Design review of the part built by this model. Coordinates are the model's own, in mm. Face numbers are marked on the shaded views. A direction names the side the tool comes from. Coordinates: 2 decimals unless noted, no trailing zeros. Write each loop counter-clockwise with the first axis right and the second up, starting at its lowest first coordinate (ties: lowest second). Pieces come first, ordered by that corner, then holes. Notation, with made-up numbers: (42, -0.5) -> (61, -0.5) arc R27 cw to (61, 21.5) -> close; hole circle Ø3 at (74.5, 35). An arc over 180 degrees is marked (long way). Return JSON: item names as keys, results as strings. Group by question number.
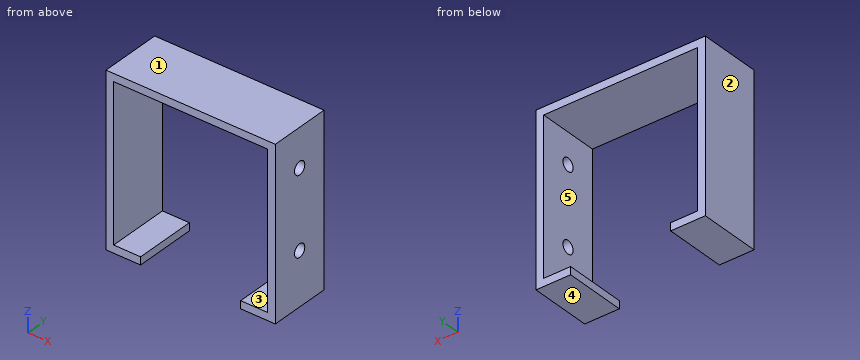
from build123d import *

# Parameters (mm, degrees)
BOSS_EXTRUDE1_DEPTH = 25.4
CUT_EXTRUDE1_REACH  = 71.85
SKETCH2_R           = 2.667


with BuildPart() as part:
    # Sketch1 → Boss-Extrude1 (new body)
    with BuildSketch(Plane(origin=(0, 0, 0), x_dir=(1, 0, 0), z_dir=(0, 1, 0))):
        Polygon((-3.175, -3.175), (-3.175, 63.5), (-3.175, 66.675), (11.1125, 66.675), (11.1125, 63.5), (0, 63.5), (0, 0), (63.5, 0), (63.5, 63.5), (52.3875, 63.5), (52.3875, 66.675), (66.675, 66.675), (66.675, 63.5), (66.675, -3.175), align=None)
    extrude(amount=BOSS_EXTRUDE1_DEPTH)

    # Sketch2 → Cut-Extrude1 (cut, up to next)
    with BuildSketch(Plane(origin=(66.675, 0, 0), x_dir=(0, 0, -1), z_dir=(1, 0, 0)), mode=Mode.PRIVATE) as cut_extrude1_sk1:
        with Locations((12.7, 12.7)):
            Circle(SKETCH2_R)
    cut_extrude1_tool1 = extrude(cut_extrude1_sk1.sketch, amount=-CUT_EXTRUDE1_REACH, mode=Mode.PRIVATE) & part.part
    add(cut_extrude1_tool1.solids().sort_by_distance((66.675, 12.7, -12.7))[0], mode=Mode.SUBTRACT)
    # Sketch2 → Cut-Extrude1 (cut, up to next)
    with BuildSketch(Plane(origin=(66.675, 0, 0), x_dir=(0, 0, -1), z_dir=(1, 0, 0)), mode=Mode.PRIVATE) as cut_extrude1_sk2:
        with Locations((44.7675, 12.7)):
            Circle(SKETCH2_R)
    cut_extrude1_tool2 = extrude(cut_extrude1_sk2.sketch, amount=-CUT_EXTRUDE1_REACH, mode=Mode.PRIVATE) & part.part
    add(cut_extrude1_tool2.solids().sort_by_distance((66.675, 12.7, -44.7675))[0], mode=Mode.SUBTRACT)


solid = part.part
Q1. For P1, Ø1.5, axis at x = 44, y = 20.5, coming from the -Z side, flat-tipped, find the tip position at first contact; note if it passes through.
Q2. For the marked faces 4 and 5, list the 3-axis set-ups (+Z, -Z, +X, -X, +Y, -Y) from which the entire face can be reached by the end or side of a thin tool; tool diameter is ignored.
Q3. We need section A-A on z = -23.5. Write out the cut boundary in (x, y) (3 decimals).
Q4. We need section C-C on y = 12.7. Write out the cut boundary in (x, z) (1 decimal), plus the area to 3 significant figures.
Q5. The part is to be moulded in two halves that separate along Z. For the marked faces 1, 2 and 3, say which applies: +Z half, -Z half, draft (parallel to the pull), parting line (faces both ways), or undercut.
Q6. We need section D-D on z = -12.7. Write out the cut boundary in (x, y) (3 decimals).
Q7. We need section B-B on x = 57. Write out the cut boundary in (y, z) (3 decimals), plus the area to 3 significant figures.
Q8. Wall thickness on L1, parallel to X at y = 14.75, z = -58 (3 decimals); L2, parallel to Z at x = 54, y = 6.75 (3 decimals); L3, parallel to Y at x = 65.45, z = -12.7: over which ranges is each line inside the solid? List them lowest first.
Findings below:
{
 "1": {"P1": "stops at z = 0"},
 "2": {"face 4": "-Z, +X, -X, +Y, -Y", "face 5": "+Y, -Y"},
 "3": {"outline": "(-3.175, 0) -> (0, 0) -> (0, 25.4) -> (-3.175, 25.4) -> close; (63.5, 0) -> (66.675, 0) -> (66.675, 25.4) -> (63.5, 25.4) -> close"},
 "4": {"outline": "(-3.2, -66.7) -> (11.1, -66.7) -> (11.1, -63.5) -> (0, -63.5) -> (0, 0) -> (63.5, 0) -> (63.5, -10) -> (66.7, -10) -> (66.7, 3.2) -> (-3.2, 3.2) -> close; (52.4, -66.7) -> (66.7, -66.7) -> (66.7, -47.4) -> (63.5, -47.4) -> (63.5, -63.5) -> (52.4, -63.5) -> close; (63.5, -42.1) -> (66.7, -42.1) -> (66.7, -15.4) -> (63.5, -15.4) -> close", "area": "682 mm^2"},
 "5": {"face 1": "+Z half", "face 2": "draft", "face 3": "undercut"},
 "6": {"outline": "(-3.175, 0) -> (0, 0) -> (0, 25.4) -> (-3.175, 25.4) -> close; (63.5, 0) -> (66.675, 0) -> (66.675, 10.033) -> (63.5, 10.033) -> close; (63.5, 15.367) -> (66.675, 15.367) -> (66.675, 25.4) -> (63.5, 25.4) -> close"},
 "7": {"outline": "(0, -66.675) -> (25.4, -66.675) -> (25.4, -63.5) -> (0, -63.5) -> close; (0, 0) -> (25.4, 0) -> (25.4, 3.175) -> (0, 3.175) -> close", "area": "161 mm^2"},
 "8": {"L1": "x = -3.175 to 0, 63.5 to 66.675", "L2": "z = -66.675 to -63.5, 0 to 3.175", "L3": "y = 0 to 10.03, 15.37 to 25.4"}
}
